```python
from build123d import *

# Parameters (mm, degrees)
BOSS_EXTRUDE1_DEPTH      = 25
BOSS_EXTRUDE1_DEPTH_BACK = 25
SKETCH1_W                = 70
SKETCH1_H                = 10
BOSS_EXTRUDE2_DEPTH      = 10
BOSS_EXTRUDE2_DEPTH_BACK = 10
CUT_EXTRUDE1_DEPTH       = 19
CUT_EXTRUDE1_DEPTH_BACK  = 16
SKETCH3_R                = 3.5
SKETCH4_W                = 50
SKETCH4_H                = 50
BOSS_EXTRUDE3_DEPTH      = 15


with BuildPart() as part:
    # Sketch1 → Boss-Extrude1 (new, two sides: drawn at the far end of the back side and taken through both)
    with BuildSketch(Plane(origin=(0, 0, 0), x_dir=(1, 0, 0), z_dir=(0, 1, 0)).offset(-BOSS_EXTRUDE1_DEPTH_BACK)):
        Rectangle(SKETCH1_W, SKETCH1_H)
    extrude(amount=BOSS_EXTRUDE1_DEPTH + BOSS_EXTRUDE1_DEPTH_BACK)

    # Sketch2 → Boss-Extrude2 (add, two sides: drawn at the far end of the back side and taken through both)
    with BuildSketch(Plane(origin=(0, 0, 0), x_dir=(1, 0, 0), z_dir=(0, 1, 0)).offset(-BOSS_EXTRUDE2_DEPTH_BACK)):
        with BuildLine():
            Line((-75, 5), (-35, 5))
            Line((-35, 5), (-35, -5))
            Line((-35, -5), (-75, -5))
            ThreePointArc((-75, -5), (-80, 0), (-75, 5))
        make_face()
    extrude(amount=BOSS_EXTRUDE2_DEPTH + BOSS_EXTRUDE2_DEPTH_BACK)

    # Sketch3 → Cut-Extrude1 (cut, two sides: drawn at the far end of the back side and taken through both)
    with BuildSketch(Plane(origin=(0, 0, 0), x_dir=(1, 0, 0), z_dir=(0, 1, 0)).offset(-CUT_EXTRUDE1_DEPTH_BACK)):
        with Locations(Location((-75.333177097, 0, 0), (0, 0, 270))):
            Circle(SKETCH3_R)
        with Locations(Location((-55, 0, 0), (0, 0, 270))):
            Circle(SKETCH3_R)
    extrude(amount=CUT_EXTRUDE1_DEPTH + CUT_EXTRUDE1_DEPTH_BACK, mode=Mode.SUBTRACT)

    # Sketch4 → Boss-Extrude3 (add)
    with BuildSketch(Plane.XY):
        with Locations((10, 0)):
            Rectangle(SKETCH4_W, SKETCH4_H)
    extrude(amount=-BOSS_EXTRUDE3_DEPTH)


solid = part.part
```
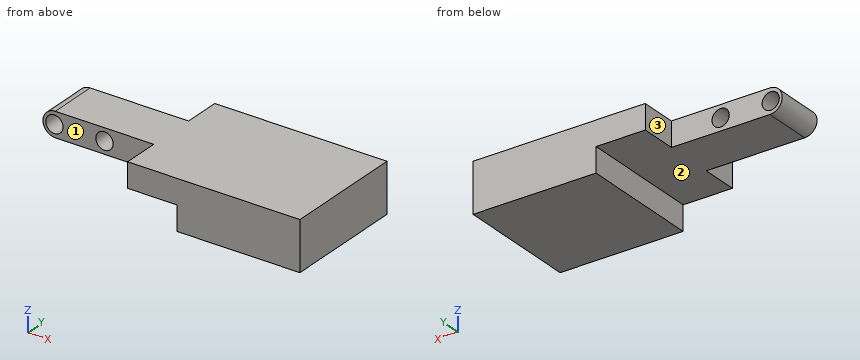
Can you work these out from the model? Positions are in its coordinate system, mm. Face numbers are marked on the shaded views. A direction names the side the tool comes from. Coordinates: 2 decimals unless noted, no trailing zeros. Loops run counter-clockwise (first coordinate to the right, second up) from the corner with the lowest first, then second, coordinate; pieces in that order, holes last.
Item 1: Suppose I cut it at A-A (z = 0). Please give me the cut outline in (x, y).
Answers below:
outline: (-80, -10) - (-78.83, -10) - (-78.83, 10) - (-80, 10) - close; (-71.83, -10) - (-58.5, -10) - (-58.5, 10) - (-71.83, 10) - close; (-51.5, -10) - (-35, -10) - (-35, -25) - (35, -25) - (35, 25) - (-35, 25) - (-35, 10) - (-51.5, 10) - close
Item 2: Suppose I cut it at B-B (x = -55). Please give me the cut outline in (y, z), then the cut area to 3 significant figures.
Answers below:
outline: (-10, -5) - (10, -5) - (10, -3.5) - (-10, -3.5) - close; (-10, 3.5) - (10, 3.5) - (10, 5) - (-10, 5) - close
area: 60.0 mm2
Item 3: Suppose I cut it at D-D (y = -4). Please give me the cut outline in (x, z).
Answers below:
outline: (-75, -5) - (-15, -5) - (-15, -15) - (35, -15) - (35, 5) - (-75, 5) arc R5 ccw to start; hole circle Ø7 at (-75.33, 0); hole circle Ø7 at (-55, 0)
Item 4: I'm going to push flat-ended pins straight in: pin 1 (8 mm diameter, centred on x = -55, z = 0, fed in from +Y); pin 2 (10 mm diameter, centred on x = -45, y = -14, fed in from -Z); pin 3 (6 mm diameter, centred on y = 11.5, z = -13, fed in from -X). Where does each tip first touch, or does it pass through?
Answers below:
pin 1: stops at y = 10
pin 2: stops at z = -5
pin 3: stops at x = -15
Item 5: Please list where these lines run through material, in increasing order: L1, parallel to X at y = -5.75, z = 0; L2, parallel to Z at x = -55, y = -1; L3, parallel to X at y = 4.5, z = -1.75.
Answers below:
L1: x = -80 to -78.83, -71.83 to -58.5, -51.5 to 35
L2: z = -5 to -3.5, 3.5 to 5
L3: x = -79.68 to -78.36, -72.3 to -58.03, -51.97 to 35
Item 6: Which directions (+Z, -Z, +X, -X, +Y, -Y) give clear straight access to the entire face, cutting with the end or side of a thin tool? Please do the marked faces 1, 2 and 3.
Answers below:
face 1: +Z, -Z, -X, -Y
face 2: -Z, -X, +Y, -Y
face 3: +Z, -Z, -X, +Y
Item 7: Suppose I cut it at C-C (y = -15.5). Please give me the cut outline in (x, z), then the cut area to 3 significant figures.
Answers below:
outline: (-35, -5) - (-15, -5) - (-15, -15) - (35, -15) - (35, 5) - (-35, 5) - close
area: 1,200 mm2
